```python
from build123d import *

# Parameters (mm, degrees)
BOSS_EXTRUDE1_DEPTH = 2.5
SKETCH2_R           = 1.5875
CUT_EXTRUDE1_DEPTH  = 23.630178965


with BuildPart() as part:
    # Sketch1 → Boss-Extrude1 (new, symmetric)
    with BuildSketch(Plane.XY):
        with BuildLine():
            Line((-18, 3.75), (18, 3.75))
            ThreePointArc((18, 3.75), (21.75, 0), (18, -3.75))
            Line((18, -3.75), (-18, -3.75))
            ThreePointArc((-18, -3.75), (-21.75, 0), (-18, 3.75))
        make_face()
    extrude(amount=BOSS_EXTRUDE1_DEPTH, both=True)

    # Sketch2 → Cut-Extrude1 (cut, through all)
    with BuildSketch(Plane.XY.offset(2.5)):
        with Locations((-18, 0)):
            Circle(SKETCH2_R)
        with Locations((18, 0)):
            Circle(SKETCH2_R)
    extrude(amount=-CUT_EXTRUDE1_DEPTH, mode=Mode.SUBTRACT)


solid = part.part
```
Geometry check sheet. Reference: the model listing, model coordinates, mm. Round coordinates to 2 decimals unless told otherwise and drop trailing zeros. Order: outer loops, then holes, each group sorted by start corner. A loop starts at its lowest first (then second) coordinate and runs counter-clockwise, first axis right, second up. Notation, with made-up numbers: (55, 45) - (104, 45) arc R25 ccw to (104, 69) - close; hole circle Ø10 at (8.25, 28). An arc over 180 degrees is marked (long way). Use a Markdown table: item, result. Add a question column.
1) Section check B-B (x = 17). Record the cut outline in (y, z), then the cut area to 3 significant figures.
2) Section check C-C (z = -1.4). Count the separate pieces of the cut face and the enclosed holes in it, then the cut area to 3 significant figures.
3) Thickness scan on line 1 along X through (y, z) = (-0.5, 1.75); line 2 along Y through (x, z) = (18, 1.6); line 3 along X through (y, z) = (-1.75, 1.85). Record the ranges inside material, lowest first.
4) Gauge pin test, flat ends, axial feed: P1, Ø2, axis at y = 1.5, z = -2, coming from the +X side; P2, Ø1, axis at y = -1.5, z = 1.5, coming from the +X side. Record the tip position at first contact, or that the pin passes through.
5) Mould release check, pull along X, two halves, no side actions. Record for faces 1 (the flat face through (0, 0, 2.5)), 2 (the cylindrical face through (19.514, 0.477, 0.035)), 3 (the cylindrical face through (21.75, 0.08, 0.04)): released by +X, released by -X, zero draft, split by the parting line, or undercut.
6) Section check A-A (y = 0). Record the cut outline in (x, z).
7) Section check D-D (y = 3.25). Record the cut outline in (x, z).
Established:
| question | item | result |
|---|---|---|
| 1 | outline | (-3.75, -2.5) - (-1.23, -2.5) - (-1.23, 2.5) - (-3.75, 2.5) - close; (1.23, -2.5) - (3.75, -2.5) - (3.75, 2.5) - (1.23, 2.5) - close |
| 1 | area | 25.2 mm2 |
| 2 | separate pieces | 1 |
| 2 | enclosed holes | 2 |
| 2 | area | 298 mm2 |
| 3 | line 1 | -21.72 to -19.51, -16.49 to 16.49, 19.51 to 21.72 |
| 3 | line 2 | -3.75 to -1.59, 1.59 to 3.75 |
| 3 | line 3 | -21.32 to 21.32 |
| 4 | P1 | x = 21.72 |
| 4 | P2 | x = 21.61 |
| 5 | face 1 | zero draft |
| 5 | face 2 | undercut |
| 5 | face 3 | released by +X |
| 6 | outline | (-21.75, -2.5) - (-19.59, -2.5) - (-19.59, 2.5) - (-21.75, 2.5) - close; (-16.41, -2.5) - (16.41, -2.5) - (16.41, 2.5) - (-16.41, 2.5) - close; (19.59, -2.5) - (21.75, -2.5) - (21.75, 2.5) - (19.59, 2.5) - close |
| 7 | outline | (-19.87, -2.5) - (19.87, -2.5) - (19.87, 2.5) - (-19.87, 2.5) - close |
